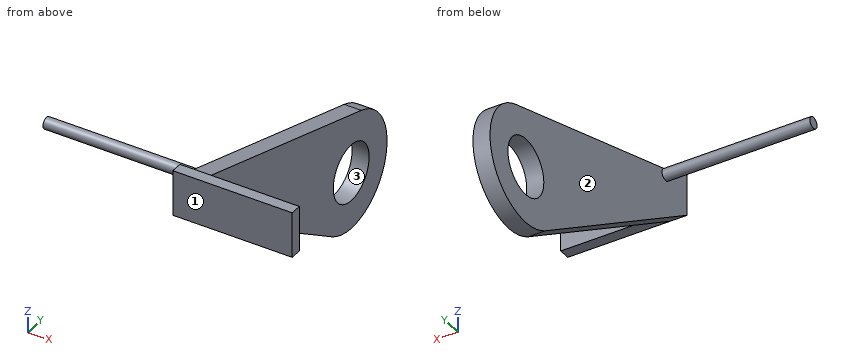
```python
from build123d import *

# Parameters (mm, degrees)
SKETCH1_W           = 2.032
SKETCH1_H           = 0.508
BOSS_EXTRUDE1_DEPTH = 5.334
SKETCH1_3_R         = 2.54
SKETCH1_3_R_2       = 1.27
BOSS_EXTRUDE2_DEPTH = 0.762
SKETCH2_R           = 0.254
BOSS_EXTRUDE3_DEPTH = 6.604


with BuildPart() as part:
    # Sketch1 → Boss-Extrude1 (new body)
    with BuildSketch(Plane(origin=(0, 0, 0), x_dir=(0, 0, -1), z_dir=(1, 0, 0))):
        with Locations((-5.334, -11.176)):
            Rectangle(SKETCH1_W, SKETCH1_H)
    extrude(amount=BOSS_EXTRUDE1_DEPTH)

    # Sketch1_3 → Boss-Extrude2 (add)
    # profile 1 of 2: a face of its own
    with BuildSketch(Plane(origin=(0, 0, 0), x_dir=(0, 0, -1), z_dir=(1, 0, 0))):
        with BuildLine():
            Line((-4.318, -11.43), (2.137587014, -1.371977316))
            ThreePointArc((2.137587014, -1.371977316), (-1.053360752, -2.311283437), (-2.437803052, 0.713243493))
            Line((-2.437803052, 0.713243493), (-5.842, -10.922))
            Line((-5.842, -10.922), (-4.318, -10.922))
            Line((-4.318, -10.922), (-4.318, -11.43))
        make_face()
    # profile 2 of 2: a face of its own
    with BuildSketch(Plane(origin=(0, 0, 0), x_dir=(0, 0, -1), z_dir=(1, 0, 0))):
        Circle(SKETCH1_3_R)
        with Locations(Location((0, 0, 0), (0, 0, 180))):
            Circle(SKETCH1_3_R_2, mode=Mode.SUBTRACT)
    extrude(amount=BOSS_EXTRUDE2_DEPTH)

    # Sketch2 → Boss-Extrude3 (add)
    with BuildSketch(Plane.ZY):
        with Locations(Location((5.27681031, -9.894775555, 0), (0, 0, 16.308227118))):
            Circle(SKETCH2_R)
    extrude(amount=BOSS_EXTRUDE3_DEPTH)


solid = part.part
```
Geometry check sheet. Reference: the model listing, model coordinates, mm. Face numbers are marked on the shaded views. Coordinates: 2 decimals unless noted, no trailing zeros. Write each loop counter-clockwise with the first axis right and the second up, starting at its lowest first coordinate (ties: lowest second). Pieces come first, ordered by that corner, then holes. Notation, with made-up numbers: (17, 86) -> (46, 86) arc R19 ccw to (46, 105) -> close; hole circle Ø6 at (-21.5, -5.5). An arc over 180 degrees is marked (long way). Use CSV: the item, a comma, the result in double quotes. Start each with the question number.
Item 1: Thickness scan on line 1 (X direction, y = -3, z = -0.25); line 2 (Y direction, x = 0.65, z = 0). Record the ranges inside material, lowest first.
Item 2: Depth check by flat-ended pin: pin 1 Ø1.5 at (x, z) = (-2.5, 3) entering from -Y; pin 2 Ø1.6 at (x, z) = (3.5, 5.5) entering from +Y; pin 3 Ø2 at (y, z) = (-5.5, 1.5) entering from +X; pin 4 Ø4.5 at (y, z) = (-6.5, 2.5) entering from -X. Enter the tip coordinate at first touch or a pass-through.
Item 3: Cross-section at D-D, the plane z = 5.25. Record the cut outline in (x, y).
Item 4: Cross-section at C-C, the plane x = 2.25. Record the cut outline in (y, z).
Item 5: Cross-section at A-A, the plane z = 0.25. Record the cut outline in (x, y), plus the area to 3 significant figures.
Item 6: Mould release check, pull along Y, two halves, no side actions. Record for the marked faces 1, 2 and 3: released by +Y, released by -Y, zero draft, split by the parting line, or undercut.
Item 7: Cross-section at B-B, the plane y = 0.25. Record the cut outline in (x, z).
Answers:
1,line 1,"0 to 0.76"
1,line 2,"-4.7 to -1.27, 1.27 to 2.54"
2,pin 1,"through"
2,pin 2,"y = -10.92"
2,pin 3,"x = 0.76"
2,pin 4,"x = 0"
3,outline,"(-6.6, -10.15) -> (0, -10.15) -> (0, -11.43) -> (5.33, -11.43) -> (5.33, -10.92) -> (0.76, -10.92) -> (0.76, -8.9) -> (0, -8.9) -> (0, -9.64) -> (-6.6, -9.64) -> close"
4,outline,"(-11.43, 4.32) -> (-10.92, 4.32) -> (-10.92, 6.35) -> (-11.43, 6.35) -> close"
5,outline,"(0, -5.09) -> (0.76, -5.09) -> (0.76, -1.25) -> (0, -1.25) -> close; (0, 1.25) -> (0.76, 1.25) -> (0.76, 2.53) -> (0, 2.53) -> close"
5,area,"3.91 mm^2"
6,face 1,"released by -Y"
6,face 2,"zero draft"
6,face 3,"undercut"
7,outline,"(0, -2.53) -> (0.76, -2.53) -> (0.76, -1.25) -> (0, -1.25) -> close; (0, 1.25) -> (0.76, 1.25) -> (0.76, 2.57) -> (0, 2.57) -> close"
